```python
from build123d import *

# Parameters (mm, degrees)
BOSS_EXTRUDE1_DEPTH = 182.6
SKETCH2_R           = 2.5
SKETCH2_R_2         = 0.85
BOSS_EXTRUDE2_DEPTH = 3
SKETCH3_R           = 3.175
CUT_EXTRUDE1_DEPTH  = 15
SKETCH4_R           = 2.6
SKETCH4_R_2         = 1.55
BOSS_EXTRUDE3_DEPTH = 6
SKETCH7_R           = 1.6
CUT_EXTRUDE3_DEPTH  = 10
SKETCH8_R           = 1.6
CUT_EXTRUDE4_DEPTH  = 10
SKETCH6_R           = 0.85
CUT_EXTRUDE2_DEPTH  = 7
SKETCH9_R           = 3.5
SKETCH9_R_2         = 1.95
BOSS_EXTRUDE4_DEPTH = 5
SKETCH10_R          = 1.6
CUT_EXTRUDE5_DEPTH  = 10
SKETCH11_W          = 23
SKETCH11_H          = 34
CUT_EXTRUDE6_DEPTH  = 10
CHAMFER1_SIZE       = 1
SKETCH12_R          = 2.65
CUT_EXTRUDE7_DEPTH  = 3.5
SKETCH13_R          = 1.05
CUT_EXTRUDE8_DEPTH  = 8
SKETCH15_R          = 1.8
CUT_EXTRUDE9_DEPTH  = 3


with BuildPart() as part:
    # Sketch1 → Boss-Extrude1 (new body)
    with BuildSketch(Plane.XY):
        Polygon((0, 5), (7.5, 8), (117.5, 8), (125, 5), (125, 0), (0, 0), align=None)
    extrude(amount=BOSS_EXTRUDE1_DEPTH)

    # Sketch2 → Boss-Extrude2 (add)
    with BuildSketch(Plane.XZ):
        with Locations((40, 173.1)):
            Circle(SKETCH2_R)
        with Locations((40, 173.1)):
            Circle(SKETCH2_R_2, mode=Mode.SUBTRACT)
        with Locations((98, 173.1)):
            Circle(SKETCH2_R)
        with Locations((98, 173.1)):
            Circle(SKETCH2_R_2, mode=Mode.SUBTRACT)
        with Locations((98, 124.1)):
            Circle(SKETCH2_R)
        with Locations((98, 124.1)):
            Circle(SKETCH2_R_2, mode=Mode.SUBTRACT)
        with Locations((40, 124.1)):
            Circle(SKETCH2_R)
        with Locations((40, 124.1)):
            Circle(SKETCH2_R_2, mode=Mode.SUBTRACT)
    extrude(amount=BOSS_EXTRUDE2_DEPTH)

    # Sketch3 → Cut-Extrude1 (cut)
    with BuildSketch(Plane(origin=(0, 8, 0), x_dir=(1, 0, 0), z_dir=(0, 1, 0))):
        with Locations((22.5, -152.6)):
            Circle(SKETCH3_R)
        with Locations((102.5, -152.6)):
            Circle(SKETCH3_R)
        with Locations((102.5, -30)):
            Circle(SKETCH3_R)
        with Locations((22.5, -30)):
            Circle(SKETCH3_R)
    extrude(amount=-CUT_EXTRUDE1_DEPTH, mode=Mode.SUBTRACT)

    # Sketch4 → Boss-Extrude3 (add)
    with BuildSketch(Plane.XZ):
        with Locations((56.15, 81.14)):
            Circle(SKETCH4_R)
        with Locations((56.15, 81.14)):
            Circle(SKETCH4_R_2, mode=Mode.SUBTRACT)
        with Locations((68.85, 81.14)):
            Circle(SKETCH4_R)
        with Locations((68.85, 81.14)):
            Circle(SKETCH4_R_2, mode=Mode.SUBTRACT)
        with Locations((68.85, 101.46)):
            Circle(SKETCH4_R)
        with Locations((68.85, 101.46)):
            Circle(SKETCH4_R_2, mode=Mode.SUBTRACT)
        with Locations((56.15, 101.46)):
            Circle(SKETCH4_R)
        with Locations((56.15, 101.46)):
            Circle(SKETCH4_R_2, mode=Mode.SUBTRACT)
    extrude(amount=BOSS_EXTRUDE3_DEPTH)

    # Sketch7 → Cut-Extrude3 (cut)
    with BuildSketch(Plane(origin=(0, 8, 0), x_dir=(1, 0, 0), z_dir=(0, 1, 0))):
        with Locations((17, -75.01)):
            Circle(SKETCH7_R)
        with Locations((17, -117.585)):
            Circle(SKETCH7_R)
        with Locations((108, -75.01)):
            Circle(SKETCH7_R)
        with Locations((108, -117.59)):
            Circle(SKETCH7_R)
    extrude(amount=-CUT_EXTRUDE3_DEPTH, mode=Mode.SUBTRACT)

    # Sketch8 → Cut-Extrude4 (cut)
    with BuildSketch(Plane(origin=(0, 8, 0), x_dir=(1, 0, 0), z_dir=(0, 1, 0))):
        with Locations((13, -141.6)):
            Circle(SKETCH8_R)
        with Locations((13, -157.6)):
            Circle(SKETCH8_R)
    extrude(amount=-CUT_EXTRUDE4_DEPTH, mode=Mode.SUBTRACT)

    # Sketch6 → Cut-Extrude2 (cut)
    with BuildSketch(Plane.XZ):
        with Locations((22.407582627, 118.246238122)):
            Circle(SKETCH6_R)
        with Locations((48.407582627, 118.246238122)):
            Circle(SKETCH6_R)
        with Locations((48.407582627, 71.246238122)):
            Circle(SKETCH6_R)
        with Locations((22.407582627, 71.246238122)):
            Circle(SKETCH6_R)
    extrude(amount=-CUT_EXTRUDE2_DEPTH, mode=Mode.SUBTRACT)

    # Sketch9 → Boss-Extrude4 (add)
    with BuildSketch(Plane.XZ):
        with Locations((117, 73)):
            Circle(SKETCH9_R)
        with Locations((117, 73)):
            Circle(SKETCH9_R_2, mode=Mode.SUBTRACT)
        with Locations((117, 8)):
            Circle(SKETCH9_R)
        with Locations((117, 8)):
            Circle(SKETCH9_R_2, mode=Mode.SUBTRACT)
        with Locations((34, 8)):
            Circle(SKETCH9_R)
        with Locations((34, 8)):
            Circle(SKETCH9_R_2, mode=Mode.SUBTRACT)
        with Locations((34, 73)):
            Circle(SKETCH9_R)
        with Locations((34, 73)):
            Circle(SKETCH9_R_2, mode=Mode.SUBTRACT)
    extrude(amount=BOSS_EXTRUDE4_DEPTH)

    # Sketch10 → Cut-Extrude5 (cut)
    with BuildSketch(Plane(origin=(0, 8, 0), x_dir=(1, 0, 0), z_dir=(0, 1, 0))):
        with Locations((32, -137.6)):
            Circle(SKETCH10_R)
        with Locations((32, -167.6)):
            Circle(SKETCH10_R)
    extrude(amount=-CUT_EXTRUDE5_DEPTH, mode=Mode.SUBTRACT)

    # Sketch11 → Cut-Extrude6 (cut)
    with BuildSketch(Plane.XZ):
        with Locations((35.407582627, 99.446238122)):
            Rectangle(SKETCH11_W, SKETCH11_H)
    extrude(amount=-CUT_EXTRUDE6_DEPTH, mode=Mode.SUBTRACT)

    # Chamfer1
    chamfer1_edges = [part.edges().sort_by_distance(p)[0] for p in [
        (35.407582627, 8, 116.446238122),
        (23.907582627, 8, 99.446238122),
        (35.407582627, 8, 82.446238122),
        (46.907582627, 8, 99.446238122),
    ]]
    chamfer(chamfer1_edges, length=CHAMFER1_SIZE)

    # Sketch12 → Cut-Extrude7 (cut)
    with BuildSketch(Plane(origin=(0, 8, 0), x_dir=(1, 0, 0), z_dir=(0, 1, 0))):
        with Locations((17, -75.01)):
            Circle(SKETCH12_R)
        with Locations((108, -75.01)):
            Circle(SKETCH12_R)
        with Locations((108, -117.59)):
            Circle(SKETCH12_R)
        with Locations((32, -137.6)):
            Circle(SKETCH12_R)
        with Locations((32, -167.6)):
            Circle(SKETCH12_R)
        with Locations((13, -157.6)):
            Circle(SKETCH12_R)
        with Locations((13, -141.6)):
            Circle(SKETCH12_R)
        with Locations((17, -117.585)):
            Circle(SKETCH12_R)
    extrude(amount=-CUT_EXTRUDE7_DEPTH, mode=Mode.SUBTRACT)

    # Sketch13 → Cut-Extrude8 (cut)
    with BuildSketch(Plane(origin=(0, 8, 0), x_dir=(1, 0, 0), z_dir=(0, 1, 0))):
        with Locations((2.5, -180.1)):
            Circle(SKETCH13_R)
        with Locations((122.5, -180.1)):
            Circle(SKETCH13_R)
        with Locations((122.5, -2.5)):
            Circle(SKETCH13_R)
        with Locations((2.5, -2.5)):
            Circle(SKETCH13_R)
    extrude(amount=-CUT_EXTRUDE8_DEPTH, mode=Mode.SUBTRACT)

    # Sketch15 → Cut-Extrude9 (cut)
    with BuildSketch(Plane(origin=(0, 8, 0), x_dir=(1, 0, 0), z_dir=(0, 1, 0))):
        with Locations((2.5, -180.1)):
            Circle(SKETCH15_R)
        with Locations((2.5, -2.5)):
            Circle(SKETCH15_R)
        with Locations((122.5, -2.5)):
            Circle(SKETCH15_R)
        with Locations((122.5, -180.1)):
            Circle(SKETCH15_R)
    extrude(amount=-CUT_EXTRUDE9_DEPTH, mode=Mode.SUBTRACT)


solid = part.part
```
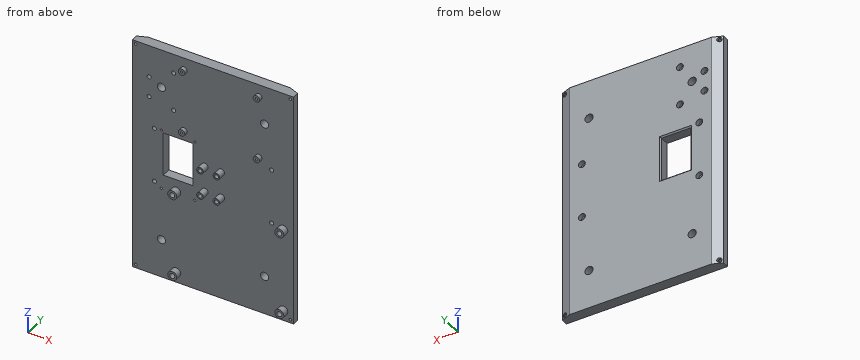
Check sheet for the modelled part. Datum: model origin and axes. Units: mm. Give positions to 0.01 mm unless a question says otherwise; leave off trailing zeros. Write each loop counter-clockwise with the first axis right and the second up, starting at its lowest first coordinate (ties: lowest second). Pieces come first, ordered by that corner, then holes. Notation, with made-up numbers: (43, 73) - (85, 73) arc R24 ccw to (85, 111) - close; hole circle Ø2 at (85.5, -10.5). An arc over 180 degrees is marked (long way). Answer as a JSON object with one key per item and string values. Group by question number.
1) Thickness scan on probe 1 along Z at (x, y) = (122.5, 5.65); probe 2 along Z at (x, y) = (17, 1.6) (3 decimals); probe 3 along Z at (x, y) = (32, 6.2). Record the ranges inside material, lowest first. Write a range as from..to.
2) Sectioned sample at B-B (z = 93). Record the cut outline in (x, y).
3) Depth check by flat-ended pin: P1, Ø1.9, axis at x = 22.5, z = 118.5, coming from the -Y side; P2, Ø2.5, axis at x = 40, z = 125, coming from the -Y side. Enter the tip coordinate at first touch or a pass-through.
4) Sectioned sample at A-A (z = 152.6). Record the cut outline in (x, y) (3 decimals).
5) Sectioned sample at C-C (y = 2.25). Give the number of separate pieces and of enclosed holes in the cut face, then the cut area to 3 significant figures.
6) Sectioned sample at D-D (z = 8). Record the cut outline in (x, y), then the cut area to 3 significant figures.
Geometry results:
{
 "1": {"probe 1": "z = 0..0.7, 4.3..178.3, 181.9..182.6", "probe 2": "z = 0..73.41, 76.61..115.985, 119.185..182.6", "probe 3": "z = 0..82.45, 116.45..134.95, 140.25..164.95, 170.25..182.6"},
 "2": {"outline": "(0, 0) - (23.91, 0) - (23.91, 7) - (22.91, 8) - (7.5, 8) - (0, 5) - close; (46.91, 0) - (125, 0) - (125, 5) - (117.5, 8) - (47.91, 8) - (46.91, 7) - close"},
 "3": {"P1": "stops at y = 0", "P2": "stops at y = -3"},
 "4": {"outline": "(0, 0) - (19.325, 0) - (19.325, 8) - (7.5, 8) - (0, 5) - close; (25.675, 0) - (99.325, 0) - (99.325, 8) - (25.675, 8) - close; (105.675, 0) - (125, 0) - (125, 5) - (117.5, 8) - (105.675, 8) - close"},
 "5": {"separate pieces": "1", "enclosed holes": "21", "area": "21,800 mm^2"},
 "6": {"outline": "(0, 0) - (30.5, 0) - (30.5, -5) - (32.05, -5) - (32.05, 0) - (35.95, 0) - (35.95, -5) - (37.5, -5) - (37.5, 0) - (113.5, 0) - (113.5, -5) - (115.05, -5) - (115.05, 0) - (118.95, 0) - (118.95, -5) - (120.5, -5) - (120.5, 0) - (125, 0) - (125, 5) - (117.5, 8) - (7.5, 8) - (0, 5) - close", "area": "1,010 mm^2"}
}
